Model file for the job. Use its own axes, mm. A direction names the side the tool comes from. Coordinates: 2 decimals unless noted, no trailing zeros. Loops run counter-clockwise (first coordinate to the right, second up) from the corner with the lowest first, then second, coordinate; pieces in that order, holes last.
from build123d import *

# Parameters (mm, degrees)
SKETCH1_W           = 33
SKETCH1_H           = 50
BOSS_EXTRUDE1_DEPTH = 2
SKETCH2_W           = 2
SKETCH2_H           = 50
BOSS_EXTRUDE2_DEPTH = 6
BOSS_EXTRUDE3_DEPTH = 6
CUT_EXTRUDE1_DEPTH  = 6


with BuildPart() as part:
    # Sketch1 → Boss-Extrude1 (new body)
    with BuildSketch(Plane(origin=(0, 0, 0), x_dir=(1, 0, 0), z_dir=(0, 1, 0))):
        with Locations((-13.079672346, -6.364652574)):
            Rectangle(SKETCH1_W, SKETCH1_H)
    extrude(amount=BOSS_EXTRUDE1_DEPTH)

    # Sketch2 → Boss-Extrude2 (add)
    with BuildSketch(Plane.XZ):
        with Locations((-28.579672346, 6.364652574)):
            Rectangle(SKETCH2_W, SKETCH2_H)
        with Locations((2.420327654, 6.364652574)):
            Rectangle(SKETCH2_W, SKETCH2_H)
    extrude(amount=BOSS_EXTRUDE2_DEPTH)

    # Sketch3 → Boss-Extrude3 (add)
    with BuildSketch(Plane(origin=(0, 2, 0), x_dir=(1, 0, 0), z_dir=(0, 1, 0))):
        Polygon((-1.456888389, -6.364652574), (-4.456888389, -6.364652574), (-7.456888389, -6.364652574), (-7.456888389, -31.364652574), (-1.456888389, -31.364652574), align=None)
        Polygon((-7.456888389, -6.364652574), (-4.456888389, -6.364652574), (-1.456888389, -6.364652574), (-1.456888389, 18.635347426), (-7.456888389, 18.635347426), align=None)
    extrude(amount=BOSS_EXTRUDE3_DEPTH)

    # Sketch4 → Cut-Extrude1 (cut)
    with BuildSketch(Plane(origin=(0, 2, 0), x_dir=(1, 0, 0), z_dir=(0, 1, 0))):
        with BuildLine():
            ThreePointArc((-10.518280368, -18.864652574), (-12.861426118, -13.207798324), (-18.518280368, -10.864652574))
            Line((-18.518280368, -10.864652574), (-18.518280368, -26.864652574))
            ThreePointArc((-18.518280368, -26.864652574), (-12.861426118, -24.521506823), (-10.518280368, -18.864652574))
        make_face()
        with BuildLine():
            Line((-18.518280368, -26.864652574), (-18.518280368, -10.864652574))
            ThreePointArc((-18.518280368, -10.864652574), (-26.518280368, -18.864652574), (-18.518280368, -26.864652574))
        make_face()
        with BuildLine():
            ThreePointArc((-18.518280368, 14.135347426), (-26.518280368, 6.135347426), (-18.518280368, -1.864652574))
            Line((-18.518280368, -1.864652574), (-18.518280368, 14.135347426))
        make_face()
        with BuildLine():
            Line((-18.518280368, 14.135347426), (-18.518280368, -1.864652574))
            ThreePointArc((-18.518280368, -1.864652574), (-12.861426118, 0.478493177), (-10.518280368, 6.135347426))
            ThreePointArc((-10.518280368, 6.135347426), (-12.861426118, 11.792201676), (-18.518280368, 14.135347426))
        make_face()
    extrude(amount=-CUT_EXTRUDE1_DEPTH, mode=Mode.SUBTRACT)


solid = part.part
Q1. Which spindle directions (+Z, -Z, +X, -X, +Y, -Y) get a long thin tool onto all of the face, cutting with end or side? Do faces 5 (the flat face through (-1.457, 5, 7)), 6 (the flat face through (-27.58, -3, 6)), 7 (the flat face through (-29, -6, 7)). Say none if no direction does.
Answers:
face 5: +Z, -Z, +X, +Y
face 6: +Z, -Z, -Y
face 7: +Z, -Z, +X, -X, -Y
Q2. Slice it at A-A (y = -3.75). List the corners of the cut face in (x, z), and give its area (3 significant figures).
Answers:
outline: (-29.58, -18.64) - (-27.58, -18.64) - (-27.58, 31.36) - (-29.58, 31.36) - close; (1.42, -18.64) - (3.42, -18.64) - (3.42, 31.36) - (1.42, 31.36) - close
area: 200 mm2
Q3. Slice it at B-B (z = 16.5). List the corners of the cut face in (x, y).
Answers:
outline: (-29.58, -6) - (-27.58, -6) - (-27.58, 0) - (-26.16, 0) - (-26.16, 2) - (-29.58, 2) - close; (-10.88, 0) - (1.42, 0) - (1.42, -6) - (3.42, -6) - (3.42, 2) - (-1.46, 2) - (-1.46, 8) - (-7.46, 8) - (-7.46, 2) - (-10.88, 2) - close
Q4. Drill centre lines: line 1 (X direction, y = -5, z = 7); line 2 (Y direction, x = -6, z = -8); line 3 (Y direction, x = -17, z = 8.5). Where is each one in solid material? Low to high.
Answers:
line 1: x = -29.58 to -27.58, 1.42 to 3.42
line 2: y = 0 to 8
line 3: y = 0 to 2
Q5. Slice it at C-C (x = -26). List the corners of the cut face in (y, z), and give its area (3 significant figures).
Answers:
outline: (0, -18.64) - (2, -18.64) - (2, -8.97) - (0, -8.97) - close; (0, -3.3) - (2, -3.3) - (2, 16.03) - (0, 16.03) - close; (0, 21.7) - (2, 21.7) - (2, 31.36) - (0, 31.36) - close
area: 77.3 mm2
Q6. Slice it at D-D (z = 5). List the corners of the cut face in (x, y), and give its area (3 significant figures).
Answers:
outline: (-29.58, -6) - (-27.58, -6) - (-27.58, 0) - (1.42, 0) - (1.42, -6) - (3.42, -6) - (3.42, 2) - (-1.46, 2) - (-1.46, 8) - (-7.46, 8) - (-7.46, 2) - (-29.58, 2) - close
area: 126 mm2
Q7. Flat gauge pins, fed straight in: P1, Ø2, axis at x = -19.5, z = 7.5, coming from the +Y side; P2, Ø14.5, axis at x = -15, z = 18, coming from the -Y side; P3, Ø5, axis at y = 3.5, z = 9, coming from the +X side; P4, Ø8, axis at y = 6.5, z = -3.5, coming from the +X side. Where does each tip first touch, or does it go through?
Answers:
P1: stops at y = 2
P2: stops at y = 0
P3: stops at x = 3.42
P4: stops at x = -1.46
Q8. Mould opens along X. For faces 1 (the flat face through (-7.457, 5, 6)), 2 (the flat face through (-19, 2, 6)), 3 (the flat face through (-10, 0, 6)), 4 (the flat face through (1.42, -3, 6)) say: +X half, -X half, draft (parallel to the pull), parting line (faces both ways), or undercut.
Answers:
face 1: -X half
face 2: draft
face 3: undercut
face 4: undercut
